```python
from build123d import *

# Parameters (mm, degrees)
SKETCH1_W                = 101.6
SKETCH1_H                = 38.1
SKETCH1_W_2              = 95.25
SKETCH1_H_2              = 31.75
BOSS_EXTRUDE1_DEPTH      = 444.5
H_0_266_DIAMETER_HOLE1_D = 6.7564
H_0_266_DIAMETER_HOLE2_D = 6.7564


with BuildPart() as part:
    # Sketch1 → Boss-Extrude1 (new body)
    with BuildSketch(Plane(origin=(0, 0, 0), x_dir=(0, 0, -1), z_dir=(1, 0, 0))):
        Rectangle(SKETCH1_W, SKETCH1_H)
        Rectangle(SKETCH1_W_2, SKETCH1_H_2, mode=Mode.SUBTRACT)
    extrude(amount=BOSS_EXTRUDE1_DEPTH)

    # H (0.266) Diameter Hole1 (through all)
    with Locations(Plane(origin=(0, 19.05, 0), x_dir=(1, 0, 0), z_dir=(0, 1, 0))):
        with Locations((25.4, 0), (63.5, 0), (349.25, 0), (425.45, 12.7), (425.45, -12.7)):
            Hole(H_0_266_DIAMETER_HOLE1_D / 2)

    # H (0.266) Diameter Hole2 (through all)
    with Locations(Plane(origin=(0, 0, -50.8), x_dir=(-1, 0, 0), z_dir=(0, 0, -1))):
        with Locations((-50.8, 0), (-374.65, 0)):
            Hole(H_0_266_DIAMETER_HOLE2_D / 2)


solid = part.part
```
The model under review builds one solid part; all positions refer to its coordinate system, in mm. A direction names the side the tool comes from. Give positions to 0.01 mm unless a question says otherwise; leave off trailing zeros. Write each loop counter-clockwise with the first axis right and the second up, starting at its lowest first coordinate (ties: lowest second). Pieces come first, ordered by that corner, then holes. Notation, with made-up numbers: (79.5, 26) - (127.5, 26) arc R21 ccw to (127.5, 44) - close; hole circle Ø2 at (12.25, 77). An arc over 180 degrees is marked (long way). Answer in a Markdown table with one row per item. Add a question column.
1. We need section A-A on z = 26.5. Write out the cut boundary in (x, y) (3 decimals).
2. Tool access review of faces 5 (the flat face through (219, -15.875, 1)), 6 (the flat face through (219, 0, 50.8)): name each direction out of +Z, -Z, +X, -X, +Y, -Y from which nothing blocks a thin tool from reaching the whole face with its end or side.
3. We need section B-B on x = 201.5. Write out the cut boundary in (y, z) (3 decimals).
4. Draft analysis for pull direction Y (two halves, no side actions). For faces 1 (the flat face through (219, 0, -50.8)), 2 (the flat face through (219, 0, -47.625)), 3 (the flat face through (219, 0, 47.625)), 4 (the flat face through (219, -19.05, 1)), state which applies: +Y half, -Y half, draft (parallel to the pull), parting line (faces both ways), or undercut.
5. Wall thickness on line 1 along Z through (x, y) = (425.45, 17.7); line 2 along Z through (x, y) = (425, -17); line 3 along Z through (x, y) = (301, -8.5) (3 decimals): over which ranges is each line inside the solid? List them lowest first. Write a range as [from, to].
6. We need section C-C on y = -7.5. Write out the cut boundary in (x, z) (3 decimals), then the cut area to 3 significant figures.
Ans:
| question | item | result |
|---|---|---|
| 1 | outline | (0, -19.05) - (444.5, -19.05) - (444.5, -15.875) - (0, -15.875) - close; (0, 15.875) - (444.5, 15.875) - (444.5, 19.05) - (0, 19.05) - close |
| 2 | face 5 | +X, -X |
| 2 | face 6 | +Z, +X, -X, +Y, -Y |
| 3 | outline | (-19.05, -50.8) - (19.05, -50.8) - (19.05, 50.8) - (-19.05, 50.8) - close; hole (-15.875, -47.625) - (15.875, -47.625) - (15.875, 47.625) - (-15.875, 47.625) - close |
| 4 | face 1 | draft |
| 4 | face 2 | undercut |
| 4 | face 3 | undercut |
| 4 | face 4 | -Y half |
| 5 | line 1 | z = [-50.8, -16.08], [-9.32, 9.32], [16.08, 50.8] |
| 5 | line 2 | z = [-50.8, -16.05], [-9.35, 9.35], [16.05, 50.8] |
| 5 | line 3 | z = [-50.8, -47.625], [47.625, 50.8] |
| 6 | outline | (0, -50.8) - (444.5, -50.8) - (444.5, -47.625) - (0, -47.625) - close; (0, 47.625) - (444.5, 47.625) - (444.5, 50.8) - (0, 50.8) - close |
| 6 | area | 2,820 mm^2 |
